Geometry: final body of the model. Coordinates: model frame, mm. Round coordinates to 2 decimals unless told otherwise and drop trailing zeros. Order: outer loops, then holes, each group sorted by start corner. A loop starts at its lowest first (then second) coordinate and runs counter-clockwise, first axis right, second up. Notation, with made-up numbers: M 30,-33.75 L 50,-33.75 A23 ccw 50,-25.75 Z; hole C 17,-28.75 d8. An arc over 180 degrees is marked long. Return JSON: item names as keys, results as strings. Group by question number.
Q1. Ray query, probe 1 along X at (y, z) = (2.4, 12.7); probe 2 along Z at (x, y) = (25, 0.7); probe 3 along Y at (x, z) = (257.3, 2.25). Return the intervals inside material, ascending.
Q2. Cut plane A-A on x = 40.5. Output: boundary loops of the cut face in (y, z) (3 decimals).
Q3. Contact query for flat-ended pins moving along their axis: pin 1 (12 mm diameter, centred on x = -134.5, z = 16.5, fed in from +Y) (3 decimals); pin 2 (1.8 mm diameter, centred on x = 25, z = 12.7, fed in from +Y); pin 3 (11 mm diameter, centred on x = -98, y = 10.5, fed in from +Z) (3 decimals). Output: stop coordinate, or through.
Q4. Cut plane B-B on y = 18.5. Output: boundary loops of the cut face in (x, z) (3 decimals).
```python
from build123d import *

# Parameters (mm, degrees)
SALIENTE_EXTRUIR1_DEPTH      = 270
SALIENTE_EXTRUIR1_DEPTH_BACK = 270
CROQUIS3_R                   = 1.5
CROQUIS3_R_2                 = 1.75
CORTAR_EXTRUIR1_DEPTH        = 3.175
CROQUIS4_R                   = 1.5
CROQUIS4_R_2                 = 1.75
CORTAR_EXTRUIR2_DEPTH        = 3.175


with BuildPart() as part:
    # Croquis1 → Saliente-Extruir1 (new body, two sides)
    with BuildSketch(Plane(origin=(0, 0, 0), x_dir=(0, 0, -1), z_dir=(1, 0, 0))) as saliente_extruir1_sk:
        Polygon((0, 25.4), (0, 0), (-25.4, 0), (-25.4, 3.175), (-3.175, 3.175), (-3.175, 25.4), align=None)
    extrude(amount=SALIENTE_EXTRUIR1_DEPTH)
    extrude(saliente_extruir1_sk.sketch, amount=-SALIENTE_EXTRUIR1_DEPTH_BACK)

    # Croquis3 → Cortar-Extruir1 (cut)
    with BuildSketch(Plane(origin=(0, 0, 0), x_dir=(-1, 0, 0), z_dir=(0, -1, 0))):
        with Locations((-25, -12.7)):
            Circle(CROQUIS3_R)
        with Locations((25, -12.7)):
            Circle(CROQUIS3_R)
        with Locations((-257.3, -12.7)):
            Circle(CROQUIS3_R_2)
        with Locations((257.3, -12.7)):
            Circle(CROQUIS3_R_2)
    extrude(amount=-CORTAR_EXTRUIR1_DEPTH, mode=Mode.SUBTRACT)

    # Croquis4 → Cortar-Extruir2 (cut)
    with BuildSketch(Plane(origin=(0, 0, 0), x_dir=(-1, 0, 0), z_dir=(0, 0, -1))):
        with Locations((25, 12.7)):
            Circle(CROQUIS4_R)
        with Locations((-25, 12.7)):
            Circle(CROQUIS4_R)
        with Locations((-257.3, 12.7)):
            Circle(CROQUIS4_R_2)
        with Locations((257.3, 12.7)):
            Circle(CROQUIS4_R_2)
    extrude(amount=-CORTAR_EXTRUIR2_DEPTH, mode=Mode.SUBTRACT)


solid = part.part
```
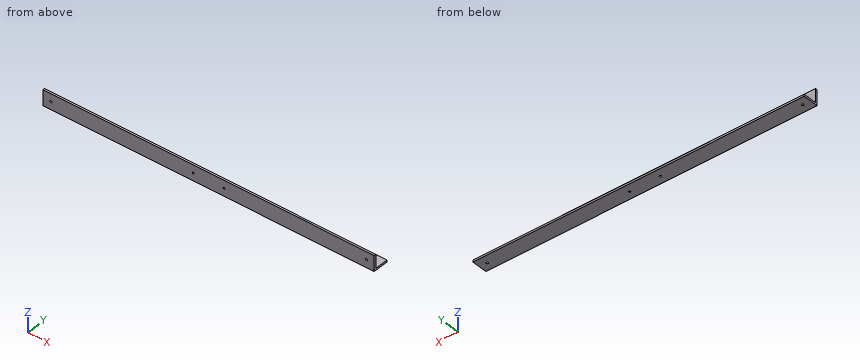
Result sheet:
{
 "1": {"probe 1": "x = -270 to -259.05, -255.55 to -26.5, -23.5 to 23.5, 26.5 to 255.55, 259.05 to 270", "probe 2": "z = 0 to 11.2, 14.2 to 25.4", "probe 3": "y = 0 to 10.95, 14.45 to 25.4"},
 "2": {"outline": "M 0,0 L 25.4,0 L 25.4,3.175 L 3.175,3.175 L 3.175,25.4 L 0,25.4 Z"},
 "3": {"pin 1": "stops at y = 3.175", "pin 2": "passes through", "pin 3": "stops at z = 3.175"},
 "4": {"outline": "M -270,0 L 270,0 L 270,3.175 L -270,3.175 Z"}
}
